Geometry: final body of the model. Coordinates: model frame, mm. Round coordinates to 2 decimals unless told otherwise and drop trailing zeros. Write each loop counter-clockwise with the first axis right and the second up, starting at its lowest first coordinate (ties: lowest second). Pieces come first, ordered by that corner, then holes. Notation, with made-up numbers: (33, -37.75) - (91, -37.75) arc R35 ccw to (91, 1.25) - close; hole circle Ø8 at (36, -18). An arc over 180 degrees is marked (long way). Write each question's results on one line, items separated by ' | '.
from build123d import *

# Parameters (mm, degrees)
SKETCH2_W           = 191
SKETCH2_H           = 136
SKETCH2_R           = 1.55
SKETCH2_R_2         = 1.549999948
SKETCH2_R_3         = 1.5
BOSS_EXTRUDE1_DEPTH = 3
SKETCH3_W           = 10
SKETCH3_H           = 3
SKETCH3_W_2         = 21
CUT_EXTRUDE1_DEPTH  = 3
SKETCH4_W           = 3
SKETCH4_H           = 10
SKETCH4_H_2         = 15
CUT_EXTRUDE2_DEPTH  = 3
CUT_EXTRUDE3_REACH  = 5
SKETCH8_R           = 5
CUT_EXTRUDE4_REACH  = 5
SKETCH9_R           = 3
CUT_EXTRUDE5_REACH  = 5
SKETCH10_R          = 1.55
CUT_EXTRUDE6_REACH  = 5
SKETCH11_R          = 1.05
SKETCH11_W          = 10
SKETCH11_H          = 12
CHAMFER1_SIZE       = 1


with BuildPart() as part:
    # Sketch2 → Boss-Extrude1 (new body)
    with BuildSketch(Plane.XY):
        with Locations((95.5, 68)):
            Rectangle(SKETCH2_W, SKETCH2_H)
        with Locations((35, 16)):
            Circle(SKETCH2_R, mode=Mode.SUBTRACT)
        with Locations((35, 10)):
            Circle(SKETCH2_R, mode=Mode.SUBTRACT)
        with Locations((24, 46.069195574)):
            Circle(SKETCH2_R, mode=Mode.SUBTRACT)
        with Locations((24, 54.069195574)):
            Circle(SKETCH2_R, mode=Mode.SUBTRACT)
        with Locations((24, 89.930804426)):
            Circle(SKETCH2_R, mode=Mode.SUBTRACT)
        with Locations((35, 120)):
            Circle(SKETCH2_R, mode=Mode.SUBTRACT)
        with Locations((35, 126)):
            Circle(SKETCH2_R, mode=Mode.SUBTRACT)
        with Locations((175.557368355, 35.25)):
            Circle(SKETCH2_R_2, mode=Mode.SUBTRACT)
        with Locations((163, 42.5)):
            Circle(SKETCH2_R_2, mode=Mode.SUBTRACT)
        with Locations((150.442631645, 35.25)):
            Circle(SKETCH2_R_2, mode=Mode.SUBTRACT)
        with Locations((150.442631645, 20.75)):
            Circle(SKETCH2_R_2, mode=Mode.SUBTRACT)
        with Locations((163, 13.5)):
            Circle(SKETCH2_R_2, mode=Mode.SUBTRACT)
        with Locations((175.557368355, 20.75)):
            Circle(SKETCH2_R_2, mode=Mode.SUBTRACT)
        with Locations((18.8, 78.5)):
            Circle(SKETCH2_R_3, mode=Mode.SUBTRACT)
        with Locations((18.8, 26)):
            Circle(SKETCH2_R_3, mode=Mode.SUBTRACT)
        with Locations((119, 73)):
            Circle(SKETCH2_R_3, mode=Mode.SUBTRACT)
        with Locations((119, 25)):
            Circle(SKETCH2_R_3, mode=Mode.SUBTRACT)
    extrude(amount=BOSS_EXTRUDE1_DEPTH)

    # Sketch3 → Cut-Extrude1 (cut)
    with BuildSketch(Plane.XY.offset(3)):
        with Locations((15, 1.5)):
            Rectangle(SKETCH3_W, SKETCH3_H)
        with Locations((35, 1.5)):
            Rectangle(SKETCH3_W, SKETCH3_H)
        with Locations((55, 1.5)):
            Rectangle(SKETCH3_W, SKETCH3_H)
        with Locations((90.5, 1.5)):
            Rectangle(SKETCH3_W_2, SKETCH3_H)
        with Locations((176, 1.5)):
            Rectangle(SKETCH3_W, SKETCH3_H)
        with Locations((156, 1.5)):
            Rectangle(SKETCH3_W, SKETCH3_H)
        with Locations((136, 1.5)):
            Rectangle(SKETCH3_W, SKETCH3_H)
    cut_extrude1 = extrude(amount=-CUT_EXTRUDE1_DEPTH, mode=Mode.SUBTRACT)

    # Mirror1: Cut-Extrude1 across plane
    add(cut_extrude1.mirror(Plane.ZX.offset(68)), mode=Mode.SUBTRACT)

    # Sketch4 → Cut-Extrude2 (cut)
    with BuildSketch(Plane.XY.offset(3)):
        with Locations((1.5, 121)):
            Rectangle(SKETCH4_W, SKETCH4_H)
        with Locations((1.5, 101)):
            Rectangle(SKETCH4_W, SKETCH4_H)
        with Locations((1.5, 81)):
            Rectangle(SKETCH4_W, SKETCH4_H)
        with Locations((1.5, 15)):
            Rectangle(SKETCH4_W, SKETCH4_H)
        with Locations((1.5, 35)):
            Rectangle(SKETCH4_W, SKETCH4_H)
        with Locations((1.5, 57.5)):
            Rectangle(SKETCH4_W, SKETCH4_H_2)
    cut_extrude2 = extrude(amount=-CUT_EXTRUDE2_DEPTH, mode=Mode.SUBTRACT)

    # Mirror2: Cut-Extrude2 across plane
    add(cut_extrude2.mirror(Plane(origin=(95.5, 0, 0), x_dir=(0, 0, 1), z_dir=(1, 0, 0))), mode=Mode.SUBTRACT)

    # Sketch8 → Cut-Extrude3 (cut, up to next)
    with BuildSketch(Plane(origin=(0, 0, 0), x_dir=(-1, 0, 0), z_dir=(0, 0, -1)), mode=Mode.PRIVATE) as cut_extrude3_sk1:
        with Locations((-163, 28)):
            Circle(SKETCH8_R)
    cut_extrude3_tool1 = extrude(cut_extrude3_sk1.sketch, amount=-CUT_EXTRUDE3_REACH, mode=Mode.PRIVATE) & part.part
    add(cut_extrude3_tool1.solids().sort_by_distance((163, 28, 0))[0], mode=Mode.SUBTRACT)

    # Sketch9 → Cut-Extrude4 (cut, up to next)
    with BuildSketch(Plane.XY.offset(3), mode=Mode.PRIVATE) as cut_extrude4_sk1:
        with Locations((85, 68)):
            Circle(SKETCH9_R)
    cut_extrude4_tool1 = extrude(cut_extrude4_sk1.sketch, amount=-CUT_EXTRUDE4_REACH, mode=Mode.PRIVATE) & part.part
    add(cut_extrude4_tool1.solids().sort_by_distance((85, 68, 3))[0], mode=Mode.SUBTRACT)

    # Sketch10 → Cut-Extrude5 (cut, up to next)
    with BuildSketch(Plane.XY.offset(3), mode=Mode.PRIVATE) as cut_extrude5_sk1:
        with Locations((61.086070947, 114.989325612)):
            Circle(SKETCH10_R)
    cut_extrude5_tool1 = extrude(cut_extrude5_sk1.sketch, amount=-CUT_EXTRUDE5_REACH, mode=Mode.PRIVATE) & part.part
    add(cut_extrude5_tool1.solids().sort_by_distance((61.086071, 114.989326, 3))[0], mode=Mode.SUBTRACT)
    # Sketch10 → Cut-Extrude5 (cut, up to next)
    with BuildSketch(Plane.XY.offset(3), mode=Mode.PRIVATE) as cut_extrude5_sk2:
        with Locations((55.342481492, 104.453141285)):
            Circle(SKETCH10_R)
    cut_extrude5_tool2 = extrude(cut_extrude5_sk2.sketch, amount=-CUT_EXTRUDE5_REACH, mode=Mode.PRIVATE) & part.part
    add(cut_extrude5_tool2.solids().sort_by_distance((55.342481, 104.453141, 3))[0], mode=Mode.SUBTRACT)
    # Sketch10 → Cut-Extrude5 (cut, up to next)
    with BuildSketch(Plane.XY.offset(3), mode=Mode.PRIVATE) as cut_extrude5_sk3:
        with Locations((138.302074071, 104.36707814)):
            Circle(SKETCH10_R)
    cut_extrude5_tool3 = extrude(cut_extrude5_sk3.sketch, amount=-CUT_EXTRUDE5_REACH, mode=Mode.PRIVATE) & part.part
    add(cut_extrude5_tool3.solids().sort_by_distance((138.302074, 104.367078, 3))[0], mode=Mode.SUBTRACT)
    # Sketch10 → Cut-Extrude5 (cut, up to next)
    with BuildSketch(Plane.XY.offset(3), mode=Mode.PRIVATE) as cut_extrude5_sk4:
        with Locations((122.038618104, 120.630534107)):
            Circle(SKETCH10_R)
    cut_extrude5_tool4 = extrude(cut_extrude5_sk4.sketch, amount=-CUT_EXTRUDE5_REACH, mode=Mode.PRIVATE) & part.part
    add(cut_extrude5_tool4.solids().sort_by_distance((122.038618, 120.630534, 3))[0], mode=Mode.SUBTRACT)
    # Sketch10 → Cut-Extrude5 (cut, up to next)
    with BuildSketch(Plane.XY.offset(3), mode=Mode.PRIVATE) as cut_extrude5_sk5:
        with Locations((64, 30)):
            Circle(SKETCH10_R)
    cut_extrude5_tool5 = extrude(cut_extrude5_sk5.sketch, amount=-CUT_EXTRUDE5_REACH, mode=Mode.PRIVATE) & part.part
    add(cut_extrude5_tool5.solids().sort_by_distance((64, 30, 3))[0], mode=Mode.SUBTRACT)
    # Sketch10 → Cut-Extrude5 (cut, up to next)
    with BuildSketch(Plane.XY.offset(3), mode=Mode.PRIVATE) as cut_extrude5_sk6:
        with Locations((46, 30)):
            Circle(SKETCH10_R)
    cut_extrude5_tool6 = extrude(cut_extrude5_sk6.sketch, amount=-CUT_EXTRUDE5_REACH, mode=Mode.PRIVATE) & part.part
    add(cut_extrude5_tool6.solids().sort_by_distance((46, 30, 3))[0], mode=Mode.SUBTRACT)
    # Sketch10 → Cut-Extrude5 (cut, up to next)
    with BuildSketch(Plane.XY.offset(3), mode=Mode.PRIVATE) as cut_extrude5_sk7:
        with Locations((137.698811825, 29.728755384)):
            Circle(SKETCH10_R)
    cut_extrude5_tool7 = extrude(cut_extrude5_sk7.sketch, amount=-CUT_EXTRUDE5_REACH, mode=Mode.PRIVATE) & part.part
    add(cut_extrude5_tool7.solids().sort_by_distance((137.698812, 29.728755, 3))[0], mode=Mode.SUBTRACT)
    # Sketch10 → Cut-Extrude5 (cut, up to next)
    with BuildSketch(Plane.XY.offset(3), mode=Mode.PRIVATE) as cut_extrude5_sk8:
        with Locations((121.435355858, 13.465299417)):
            Circle(SKETCH10_R)
    cut_extrude5_tool8 = extrude(cut_extrude5_sk8.sketch, amount=-CUT_EXTRUDE5_REACH, mode=Mode.PRIVATE) & part.part
    add(cut_extrude5_tool8.solids().sort_by_distance((121.435356, 13.465299, 3))[0], mode=Mode.SUBTRACT)

    # Sketch11 → Cut-Extrude6 (cut, up to next)
    with BuildSketch(Plane.XY.offset(3), mode=Mode.PRIVATE) as cut_extrude6_sk1:
        with Locations((143, 47.5)):
            Circle(SKETCH11_R)
    cut_extrude6_tool1 = extrude(cut_extrude6_sk1.sketch, amount=-CUT_EXTRUDE6_REACH, mode=Mode.PRIVATE) & part.part
    add(cut_extrude6_tool1.solids().sort_by_distance((143, 47.5, 3))[0], mode=Mode.SUBTRACT)
    # Sketch11 → Cut-Extrude6 (cut, up to next)
    with BuildSketch(Plane.XY.offset(3), mode=Mode.PRIVATE) as cut_extrude6_sk2:
        with Locations((140, 63.5)):
            Rectangle(SKETCH11_W, SKETCH11_H)
    cut_extrude6_tool2 = extrude(cut_extrude6_sk2.sketch, amount=-CUT_EXTRUDE6_REACH, mode=Mode.PRIVATE) & part.part
    add(cut_extrude6_tool2.solids().sort_by_distance((140, 63.5, 3))[0], mode=Mode.SUBTRACT)

    # Chamfer1
    chamfer1_edges = [part.edges().sort_by_distance(p)[0] for p in [
        (145, 69.5, 1.5),
        (145, 57.5, 1.5),
        (135, 57.5, 1.5),
        (135, 69.5, 1.5),
    ]]
    chamfer(chamfer1_edges, length=CHAMFER1_SIZE)


solid = part.part
Q1. Pin query (flat end, axial travel): pin 1 (1.5 mm diameter, centred on x = 156.5, z = 1, fed in from +Y); pin 2 (0.9 mm diameter, centred on y = 103, z = 1.5, fed in from +X); pin 3 (1.5 mm diameter, centred on x = 138.5, z = 1.5, fed in from -Y). Return the tip coordinate at first contact, or that it passes through.
Answer block:
pin 1: y = 133 | pin 2: x = 188 | pin 3: y = 3
Q2. Ray query, line 1 along Y through (x, z) = (163, 1.1); line 2 along Y through (x, z) = (143, 0.55); line 3 along Y through (x, z) = (46, 1.6). Return the intervals inside material, ascending.
Answer block:
line 1: 0 to 11.95, 15.05 to 23, 33 to 40.95, 44.05 to 136 | line 2: 0 to 46.45, 48.55 to 57.5, 69.5 to 136 | line 3: 0 to 28.45, 31.55 to 136
Q3. Mould query, pull axis X, two halves, no side actions, for faces 1 (the flat face through (94, 69, 3)), 2 (the cylindrical face through (167, 25, 1)). Classes: pulls with the +X half, pulls with the -X half, needs draft (parallel to the pull), parting line crosses it, or undercut.
Answer block:
face 1: needs draft | face 2: undercut
Q4. Section query A-A, the plane x = 85. Return loops of the section in (y, z), plus the area to 3 significant figures.
Answer block:
outline: (3, 0) - (65, 0) - (65, 3) - (3, 3) - close; (71, 0) - (133, 0) - (133, 3) - (71, 3) - close | area: 372 mm2
